Source: CAD feature listing. Evaluate the final solid. Frame: model axes, mm. A direction names the side the tool comes from. Round coordinates to 2 decimals unless told otherwise and drop trailing zeros. Loops run counter-clockwise (first coordinate to the right, second up) from the corner with the lowest first, then second, coordinate; pieces in that order, holes last.
Item 1: Pull-direction query (X, two-part tool) for faces 1 (the flat face through (353, -115, 7)), 2 (the cylindrical face through (359.438, -60.472, 11.056)), 3 (the flat face through (193, -71, 0)), 4 (the flat face through (0, -74, 7)); classes: released by +X, released by -X, zero draft, split by the parting line, or undercut.
Item 2: Section query C-C on y = -10. Return loops of the section in (x, z), then the cut area to 3 significant figures.
Item 3: Section query B-B on y = -122.5. Return loops of the section in (x, z).
Item 4: First-contact query: P1, Ø6.5, axis at x = 10, y = -135, coming from the +Z side; P2, Ø17.5, axis at x = 353, y = -107.5, coming from the -Z side. Flat tips, straight axial feed; report the tip coordinate or a pass-through.
Item 5: Section query A-A on x = 353. Return loops of the section in (y, z).
Item 6: Ray query, L1, parallel to Y at x = 353, z = 3; L2, parallel to Y at x = 353, z = 10; L3, parallel to X at y = -107.5, z = 3. Return the intervals inside material, ascending.
Item 7: Section query D-D on z = 4.5. Give the number of separate pieces and of enclosed holes in the cut face, then the cut area to 3 significant figures.
Item 8: Access query for faces 5 (the cylindrical face through (9.241, -138.417, 7.605)), 6 (the cylindrical face through (352.643, -96.506, 3.451)). Directions: +Z, -Z, +X, -X, +Y, -Y. A direction counts if a zero-diameter tool reaches every point of the face in a straight line with its end or side. Return the directions, or none.
```python
from build123d import *

# Parameters (mm, degrees)
SKIZZE1_W                                            = 380
SKIZZE1_H                                            = 145
AUFSATZ_LINEAR_AUSTRAGEN1_DEPTH                      = 15
F_7_0_7_DURCHMESSER_BOHRUNG1_D                       = 7
STIRNSENKUNG_F_R_M12_SECHSKANTSCHRAUBE_M_D           = 13.5
STIRNSENKUNG_F_R_M12_SECHSKANTSCHRAUBE_M_CBORE_D     = 22
STIRNSENKUNG_F_R_M12_SECHSKANTSCHRAUBE_M_CBORE_DEPTH = 7
LINEARES_MUSTER1_COUNT                               = 2
LINEARES_MUSTER1_PITCH                               = 15


with BuildPart() as part:
    # Skizze1 → Aufsatz-Linear austragen1 (new body)
    with BuildSketch(Plane(origin=(0, 0, 0), x_dir=(-1, 0, 0), z_dir=(0, 0, -1))):
        with Locations((-190, -72.5)):
            Rectangle(SKIZZE1_W, SKIZZE1_H)
    extrude(amount=-AUFSATZ_LINEAR_AUSTRAGEN1_DEPTH)

    # Ø7.0 (7) Durchmesser Bohrung1 (through all)
    with Locations(Plane(origin=(0, 0, 0), x_dir=(-1, 0, 0), z_dir=(0, 0, -1))):
        with Locations((-10, -135), (-10, -10), (-285, -10), (-285, -135)):
            Hole(F_7_0_7_DURCHMESSER_BOHRUNG1_D / 2)

    # Stirnsenkung für M12 Sechskantschraube mit Schaft1 (through all)
    with Locations(Plane(origin=(0, 0, 0), x_dir=(-1, 0, 0), z_dir=(0, 0, -1))):
        with Locations((-63, -62.5), (-63, -107.5), (-353, -107.5), (-353, -62.5)):
            stirnsenkung_f_r_m12_sechskantschraube_m = CounterBoreHole(STIRNSENKUNG_F_R_M12_SECHSKANTSCHRAUBE_M_D / 2, STIRNSENKUNG_F_R_M12_SECHSKANTSCHRAUBE_M_CBORE_D / 2, STIRNSENKUNG_F_R_M12_SECHSKANTSCHRAUBE_M_CBORE_DEPTH)

    # Lineares Muster1: Stirnsenkung für M12 Sechskantschraube mit Schaft1 ×2
    with Locations(*[(0, -i * LINEARES_MUSTER1_PITCH, 0) for i in range(1, LINEARES_MUSTER1_COUNT)]):
        add(stirnsenkung_f_r_m12_sechskantschraube_m, mode=Mode.SUBTRACT)


solid = part.part
```
Data:
1. face 1: undercut
1. face 2: undercut
1. face 3: zero draft
1. face 4: released by -X
2. outline: (0, 0) - (6.5, 0) - (6.5, 15) - (0, 15) - close; (13.5, 0) - (281.5, 0) - (281.5, 15) - (13.5, 15) - close; (288.5, 0) - (380, 0) - (380, 15) - (288.5, 15) - close
2. area: 5,490 mm2
3. outline: (0, 0) - (52, 0) - (52, 7) - (56.25, 7) - (56.25, 15) - (0, 15) - close; (69.75, 7) - (74, 7) - (74, 0) - (342, 0) - (342, 7) - (346.25, 7) - (346.25, 15) - (69.75, 15) - close; (359.75, 7) - (364, 7) - (364, 0) - (380, 0) - (380, 15) - (359.75, 15) - close
4. P1: passes through
4. P2: stops at z = 7
5. outline: (-145, 0) - (-133.5, 0) - (-133.5, 7) - (-129.25, 7) - (-129.25, 15) - (-145, 15) - close; (-115.75, 7) - (-114.25, 7) - (-114.25, 15) - (-115.75, 15) - close; (-100.75, 7) - (-96.5, 7) - (-96.5, 0) - (-88.5, 0) - (-88.5, 7) - (-84.25, 7) - (-84.25, 15) - (-100.75, 15) - close; (-70.75, 7) - (-69.25, 7) - (-69.25, 15) - (-70.75, 15) - close; (-55.75, 7) - (-51.5, 7) - (-51.5, 0) - (0, 0) - (0, 15) - (-55.75, 15) - close
6. L1: y = -145 to -133.5, -96.5 to -88.5, -51.5 to 0
6. L2: y = -145 to -129.25, -115.75 to -114.25, -100.75 to -84.25, -70.75 to -69.25, -55.75 to 0
6. L3: x = 0 to 52, 74 to 342, 364 to 380
7. separate pieces: 1
7. enclosed holes: 8
7. area: 52,200 mm2
8. face 5: +Z, -Z
8. face 6: -Z
